from build123d import *

# Parameters (mm, degrees)
F0_W     = 70
F0_H     = 70
F1_DEPTH = 100
F2_SIZE  = 5
F3_W     = 70
F3_H     = 70
F4_DEPTH = 2295
F5_R     = 6
F6_DEPTH = 70.001


with BuildPart() as f1:
    # F0 (on Top) → F1 (new body)
    with BuildSketch(Plane.XY):
        Rectangle(F0_W, F0_H)
    extrude(amount=F1_DEPTH)

    # F2
    f2_edges = [f1.edges().sort_by_distance(p)[0] for p in [
        (-35, -35, 50),
        (35, -35, 50),
        (35, 35, 50),
        (-35, 35, 50),
    ]]
    chamfer(f2_edges, length=F2_SIZE)

    # F3 (on face) → F4 (join)
    with BuildSketch(Plane.XY.offset(100)):
        Rectangle(F3_W, F3_H)
    extrude(amount=F4_DEPTH)

    # F5 (on face) → F6 (cut, through all)
    with BuildSketch(Plane.YZ.offset(35)):
        with Locations((0, 40)):
            Circle(F5_R)
        Polygon((35, 2395), (-35, 2395), (35, 2371.666667), align=None)
    extrude(amount=-F6_DEPTH, mode=Mode.SUBTRACT)


solid = f1.part
Verification items for the finished model (mm, model axes). Round coordinates to 2 decimals unless told otherwise and drop trailing zeros. Write item = value, one per line.
Q1. Material ranges on L1, parallel to Z at x = -10.5, y = 0; L2, parallel to Z at x = 25, y = -2; L3, parallel to Z at x = 7.5, y = 7, recorded low to high.
Here are the results:
L1 = 0 to 34, 46 to 2383.33
L2 = 0 to 34.34, 45.66 to 2384
L3 = 0 to 2381
Q2. Mould release check, pull along X, two halves, no side actions. Record for faces 1 (the flat face through (0.5, -0.5, 2383.5)), 2 (the flat face through (-35, 0, 1181)), 3 (the flat face through (35, 0, 1181)): +X half, -X half, draft (parallel to the pull), parting line (faces both ways), or undercut.
Here are the results:
face_1 = draft
face_2 = -X half
face_3 = +X half
Q3. Depth check by flat-ended pin: pin 1 (2 mm diameter, centred on x = -3.5, y = -18, fed in from +Z); pin 2 (5 mm diameter, centred on x = -26.5, y = 24.5, fed in from +Z); pin 3 (1.5 mm diameter, centred on x = 33, y = 33, fed in from -Z); pin 4 (1 mm diameter, centred on x = -20, y = 13.5, fed in from +Z). Enter the tip coordinate at first touch or a pass-through.
Here are the results:
pin_1 = 2389.67
pin_2 = 2376
pin_3 = 0
pin_4 = 2379
